from build123d import *

# Parameters (mm, degrees)
BOSS_EXTRUDE1_DEPTH = 5
FILLET1_R           = 10
SKETCH2_R           = 1.375
SKETCH2_R_2         = 3.75
CUT_EXTRUDE1_DEPTH  = 116.680049132
SKETCH3_R           = 1.25
SKETCH3_W           = 14
SKETCH3_H           = 20
CUT_EXTRUDE2_DEPTH  = 5
SKETCH5_R           = 30.5
SKETCH5_R_2         = 27.5
BOSS_EXTRUDE2_DEPTH = 24
FILLET2_START       = 5
FILLET2_2_OUTLINE_R = 1.375
FILLET2_2_DEPTH     = 4.125417965
FILLET3_R           = 10


with BuildPart() as part:
    # Sketch1 → Boss-Extrude1 (new body)
    with BuildSketch(Plane(origin=(0, 0, 0), x_dir=(1, 0, 0), z_dir=(0, 1, 0))):
        Polygon((-43.18, 0), (43.18, 0), (43.18, -28), (59, -55.467430874), (59, -99.377430874), (-59, -99.377430874), (-59, -55.467430874), (-43.18, -28), align=None)
    extrude(amount=BOSS_EXTRUDE1_DEPTH)

    # Fillet1
    fillet1_edges = [part.edges().sort_by_distance(p)[0] for p in [
        (-43.18, 2.5, 0),
        (43.18, 2.5, 0),
    ]]
    fillet(fillet1_edges, radius=FILLET1_R)

    # Sketch2 → Cut-Extrude1 (cut, through all)
    with BuildSketch(Plane(origin=(0, 5, 0), x_dir=(1, 0, 0), z_dir=(0, 1, 0))):
        with Locations(Location((-51.25, -93.627430874, 0), (0, 0, 270))):
            Circle(SKETCH2_R)
        with Locations(Location((-35.43, -7.75, 0), (0, 0, 270))):
            Circle(SKETCH2_R)
        with Locations(Location((35.43, -7.75, 0), (0, 0, 270))):
            Circle(SKETCH2_R)
        with Locations(Location((51.25, -93.627430874, 0), (0, 0, 270))):
            Circle(SKETCH2_R)
        with Locations((-59, -55.467430874)):
            Circle(SKETCH2_R_2)
        with Locations((-43.18, -28)):
            Circle(SKETCH2_R_2)
        with Locations((43.18, -28)):
            Circle(SKETCH2_R_2)
        with Locations((59, -55.467430874)):
            Circle(SKETCH2_R_2)
    extrude(amount=-CUT_EXTRUDE1_DEPTH, mode=Mode.SUBTRACT)

    # Sketch3 → Cut-Extrude2 (cut)
    with BuildSketch(Plane(origin=(0, 5, 0), x_dir=(1, 0, 0), z_dir=(0, 1, 0))):
        with Locations(Location((-15, -35.859343003, 0), (0, 0, 270))):
            Circle(SKETCH3_R)
        with Locations(Location((15, -35.859343003, 0), (0, 0, 270))):
            Circle(SKETCH3_R)
        with Locations(Location((15, -65.859343003, 0), (0, 0, 270))):
            Circle(SKETCH3_R)
        with Locations(Location((-15, -65.859343003, 0), (0, 0, 270))):
            Circle(SKETCH3_R)
        with Locations((0, -65)):
            Rectangle(SKETCH3_W, SKETCH3_H)
    extrude(amount=-CUT_EXTRUDE2_DEPTH, mode=Mode.SUBTRACT)

    # Sketch5 → Boss-Extrude2 (add)
    with BuildSketch(Plane(origin=(0, 5, 0), x_dir=(1, 0, 0), z_dir=(0, 1, 0))):
        with Locations(Location((0, -50, 0), (0, 0, 90))):
            Circle(SKETCH5_R)
        with Locations(Location((0, -50, 0), (0, 0, 270))):
            Circle(SKETCH5_R_2, mode=Mode.SUBTRACT)
    extrude(amount=BOSS_EXTRUDE2_DEPTH)

    # Fillet2: read off the stored shape, not the designer's step
    # Fillet2 outline → Fillet2 (revolve)
    with BuildSketch(Plane.XY.offset(50)):
        with BuildLine():
            Line((30.5, 5), (59.893876913, 5))
            ThreePointArc((59.893876913, 5), (40.920210952, 11.762099923), (30.5, 29))
            Line((30.5, 29), (30.5, 5))
        make_face()
    revolve(axis=Axis((0, 0, 50), (0, 1, 0)))

    # Fillet2 2 outline → Fillet2 2 (cut)
    with BuildSketch(Plane(origin=(0, 0, 0), x_dir=(1, 0, 0), z_dir=(0, 1, 0)).offset(FILLET2_START)):
        with Locations((35.43, -7.75)):
            Circle(FILLET2_2_OUTLINE_R)
        with Locations((-35.43, -7.75)):
            Circle(FILLET2_2_OUTLINE_R)
        with BuildLine():
            Line((33.899053261, -99.377430874), (-33.899053261, -99.377430874))
            ThreePointArc((-33.899053261, -99.377430874), (0, -109.893876913), (33.899053261, -99.377430874))
        make_face()
        with BuildLine():
            ThreePointArc((-43.043276128, -8.352036402), (-57.254609777, -32.416310088), (-59, -60.309049019))
            Line((-59, -60.309049019), (-59, -59.217430874))
            ThreePointArc((-59, -59.217430874), (-55.377270458, -56.436105569), (-57.128401901, -52.217873895))
            Line((-57.128401901, -52.217873895), (-45.051598099, -31.249556979))
            ThreePointArc((-45.051598099, -31.249556979), (-39.557270458, -28.968674695), (-43.18, -24.25))
            Line((-43.18, -24.25), (-43.18, -10))
            ThreePointArc((-43.18, -10), (-43.145760415, -9.173187229), (-43.043276128, -8.352036402))
        make_face()
        with BuildLine():
            ThreePointArc((32.973875897, 0), (0, 9.893876913), (-32.973875897, 0))
            Line((-32.973875897, 0), (32.973875897, 0))
        make_face()
        with BuildLine():
            ThreePointArc((59, -60.309049019), (57.254609777, -32.416310088), (43.043276128, -8.352036402))
            ThreePointArc((43.043276128, -8.352036402), (43.145760415, -9.173187229), (43.18, -10))
            Line((43.18, -10), (43.18, -24.25))
            ThreePointArc((43.18, -24.25), (39.557270458, -28.968674695), (45.051598099, -31.249556979))
            Line((45.051598099, -31.249556979), (57.128401901, -52.217873895))
            ThreePointArc((57.128401901, -52.217873895), (55.377270458, -56.436105569), (59, -59.217430874))
            Line((59, -59.217430874), (59, -60.309049019))
        make_face()
    extrude(amount=FILLET2_2_DEPTH, mode=Mode.SUBTRACT)

    # Fillet3
    fillet3_edges = [part.edges().sort_by_distance(p)[0] for p in [
        (59, 2.5, 99.377430874),
        (-59, 2.5, 99.377430874),
    ]]
    fillet(fillet3_edges, radius=FILLET3_R)


solid = part.part
Could you check a few things on this model? Use its own coordinates, in mm. A direction names the side the tool comes from. Give positions to 0.01 mm unless a question says otherwise; leave off trailing zeros. Write each loop counter-clockwise with the first axis right and the second up, starting at its lowest first coordinate (ties: lowest second). Pieces come first, ordered by that corner, then holes. Notation, with made-up numbers: (13.5, 6) -> (63.5, 6) arc R33 cw to (63.5, 38) -> close; hole circle Ø10 at (4, -20). An arc over 180 degrees is marked (long way). Answer as CSV lines item,"result". Start each with the question number.
(1) If we section it at B-B, the plane y = 2.5: Give the number of separate pieces and of enclosed holes in the cut face, and give its area (3 significant figures).
(2) Please list where these lines run through material, in increasing order: line 1 (X direction, y = 1.1, z = 7.75) (3 decimals); line 2 (Y direction, x = -22.5, z = 44); line 3 (X direction, y = 2, z = 13.5).
(3) If we section it at C-C, the plane y = 27: Write out the boundary of the cut face in (x, z), and give its area (3 significant figures).
(4) If we section it at D-D, the plane y = 12.5: Write out the boundary of the cut face in (x, z).
(5) If we mould it in two halves opening along Z, with no side actions, what happens to faces 1 (the face through (-55.99, 2.54, 96.53)), 2 (the face through (-51, 5, 88)), 3 (the face through (0, 3, 0)), 4 (the face through (0, 3, 75))? For each: +Z half, -Z half, draft (parallel to the pull), parting line (faces both ways), or undercut.
(6) Which directions (+Z, -Z, +X, -X, +Y, -Y) give clear straight access to the entire face, cutting with the end or side of a thin tool? Please do faces 5 (the face through (43.18, 3, 17)), 6 (the face through (-16.733, 16.832, 28.177)), 7 (the face through (0, 3, 55)).
(7) If we section it at A-A, the plane x = 0: Write out the boundary of the cut face in (y, z).
(8) I'm going to push flat-ended pins straight in: pin 1 Ø9 at (x, z) = (-36, 5) entering from +Y; pin 2 Ø3.5 at (y, z) = (1.5, 20) entering from +X; pin 3 Ø5 at (y, z) = (22, 72) entering from -X. Where does each tip first touch, or does it pass through?
Answer list:
1,separate pieces,"1"
1,enclosed holes,"9"
1,area,"9,910 mm^2"
2,line 1,"-42.924 to -36.805, -34.055 to 34.055, 36.805 to 42.924"
2,line 2,"0 to 5"
2,line 3,"-43.18 to 43.18"
3,outline,"circle Ø61.96 at (0, 50); hole circle Ø55 at (0, 50)"
3,area,"639 mm^2"
4,outline,"circle Ø80.1 at (0, 50); hole circle Ø55 at (0, 50)"
5,face 1,"+Z half"
5,face 2,"draft"
5,face 3,"-Z half"
5,face 4,"undercut"
6,face 5,"-Z, +X, +Y, -Y"
6,face 6,"+Y"
6,face 7,"+Y, -Y"
7,outline,"(0, 0) -> (6.68, 0) arc R30 cw to (29, 19.5) -> (29, 22.5) -> (5, 22.5) -> (5, 55) -> (0, 55) -> close; (0, 75) -> (5, 75) -> (5, 77.5) -> (29, 77.5) -> (29, 80.5) arc R30 cw to (6.9, 99.38) -> (0, 99.38) -> close"
8,pin 1,"y = 5.77"
8,pin 2,"x = 43.18"
8,pin 3,"x = -27.05"
